For this review, take the finished solid that the model builds, in its own axes (mm). A direction names the side the tool comes from. Coordinates: 2 decimals unless noted, no trailing zeros. Order: outer loops, then holes, each group sorted by start corner. A loop starts at its lowest first (then second) coordinate and runs counter-clockwise, first axis right, second up. Notation, with made-up numbers: (76, 87) -> (115, 87) arc R23 cw to (115, 126) -> close; hole circle Ø9 at (44, 50). An arc over 180 degrees is marked (long way). Answer as a JSON object with one key per item and string values. Group by question number.
1) Draft analysis for pull direction X (two halves, no side actions). For faces 1 (the flat face through (790, -45, 250)), 2 (the cylindrical face through (-934.65, -36.38, 265.58)), 3 (the flat face through (-1130, -129, 25)), state which applies: +X half, -X half, draft (parallel to the pull), parting line (faces both ways), or undercut.
2) For pin 1 (23 mm diameter, centred on x = 1335, z = 424.71, fed in from +Y); pin 2 (15 mm diameter, centred on y = -172.5, z = 35, fed in from +X); pin 3 (10 mm diameter, centred on x = 96, y = -20.5, fed in from -Z); pin 4 (15 mm diameter, centred on y = -78, z = 15.5, fed in from -X), all flat-tipped, find the tip position at first contact; note any pin that passes through.
3) Add section A-A, the plane y = -141.5. Write out the cut boundary in (x, z).
4) Wall thickness on L1, parallel to Z at x = 1335, y = -260.25; L2, parallel to Y at x = 1092.5, z = 32; L3, parallel to Z at x = -1175, y = -262.25: over which ranges is each line inside the solid? List them lowest first.
5) Machinability: for faces 4 (the flat face through (1130, -126, 25)), 5 (the cylindrical face through (795.924, -31.007, 137.576)), 6 (the flat face through (1100, -154, 25)), 7 (the flat face through (-960, -45, 250)), 8 (the flat face through (-910, -45, 250)), which of the approach directions +Z, -Z, +X, -X, +Y, -Y give a long, thin tool a straight path to every point of the face, cutting with its end or side? Answer none if there is none.
6) Add section C-C, the plane x = -526. Write out the cut boundary in (y, z), then the cut area to 3 significant figures.
7) Add section B-B, the plane z = 168. Write out the cut boundary in (x, y).
from build123d import *

# Parameters (mm, degrees)
BOSS_EXTRUDE1_DEPTH = 50
SKETCH2_W           = 200
SKETCH2_H           = 20
BOSS_EXTRUDE2_DEPTH = 500
SKETCH4_R           = 20
BOSS_EXTRUDE3_DEPTH = 200
SKETCH6_R           = 30
SKETCH6_R_2         = 12
BOSS_EXTRUDE4_DEPTH = 25
SKETCH8_W           = 350
SKETCH8_H           = 20
BOSS_EXTRUDE5_DEPTH = 500
SKETCH9_R           = 20
CUT_EXTRUDE1_DEPTH  = 2356.175152722
LPATTERN2_COUNT     = 2
LPATTERN2_PITCH     = 1750
LPATTERN4_COUNT     = 2
LPATTERN4_PITCH     = 120
LPATTERN5_COUNT     = 2
LPATTERN5_PITCH     = 1600
CUT_EXTRUDE2_REACH  = 1488.01
SKETCH10_R          = 10
SKETCH11_R          = 10
CUT_EXTRUDE3_DEPTH  = 40


with BuildPart() as part:
    # Sketch1 → Boss-Extrude1 (new body)
    with BuildSketch(Plane.XY):
        Polygon((-1130, 0), (1130, 0), (1130, -255), (1100, -255), (1100, -50), (-1100, -50), (-1100, -255), (-1130, -255), align=None)
    extrude(amount=BOSS_EXTRUDE1_DEPTH)

    # Sketch2 → Boss-Extrude2 (add)
    with BuildSketch(Plane.XY):
        with Locations((-1125, -265)):
            Rectangle(SKETCH2_W, SKETCH2_H)
    extrude(amount=BOSS_EXTRUDE2_DEPTH)

    # Sketch4 → Boss-Extrude3 (add)
    with BuildSketch(Plane.XY.offset(50)):
        with Locations(Location((-935, -25, 0), (0, 0, 180))):
            Circle(SKETCH4_R)
    boss_extrude3 = extrude(amount=BOSS_EXTRUDE3_DEPTH)

    # Sketch6 → Boss-Extrude4 (add, symmetric)
    with BuildSketch(Plane(origin=(-935, 0, 0), x_dir=(0, -1, 0), z_dir=(-1, 0, 0))):
        with Locations(Location((25, 250, 0), (0, 0, 90))):
            Circle(SKETCH6_R)
        with Locations(Location((25, 250, 0), (0, 0, 90))):
            Circle(SKETCH6_R_2, mode=Mode.SUBTRACT)
    boss_extrude4 = extrude(amount=BOSS_EXTRUDE4_DEPTH, both=True)

    # Sketch8 → Boss-Extrude5 (add)
    with BuildSketch(Plane(origin=(0, 0, 0), x_dir=(-1, 0, 0), z_dir=(0, 0, -1))):
        with Locations((-1200, -265)):
            Rectangle(SKETCH8_W, SKETCH8_H)
    extrude(amount=-BOSS_EXTRUDE5_DEPTH)

    # Sketch9 → Cut-Extrude1 (cut, through all)
    with BuildSketch(Plane(origin=(-910, 0, 0), x_dir=(0, 0, -1), z_dir=(1, 0, 0))):
        with Locations((-249.707622987, -24.214075722)):
            Circle(SKETCH9_R)
    cut_extrude1 = extrude(amount=-CUT_EXTRUDE1_DEPTH, mode=Mode.SUBTRACT)

    # LPattern2: Boss-Extrude3, Boss-Extrude4, Cut-Extrude1 ×2
    with Locations(*[(i * LPATTERN2_PITCH, 0, 0) for i in range(1, LPATTERN2_COUNT)]):
        add(boss_extrude3)
        add(boss_extrude4)
        add(cut_extrude1, mode=Mode.SUBTRACT)

    # LPattern4: Boss-Extrude3, Boss-Extrude4, Cut-Extrude1 ×2
    with Locations(*[(i * LPATTERN4_PITCH, 0, 0) for i in range(1, LPATTERN4_COUNT)]):
        add(boss_extrude3)
        add(boss_extrude4)
        add(cut_extrude1, mode=Mode.SUBTRACT)

    # LPattern5: Boss-Extrude3, Boss-Extrude4, Cut-Extrude1 ×2
    with Locations(*[(i * LPATTERN5_PITCH, 0, 0) for i in range(1, LPATTERN5_COUNT)]):
        add(boss_extrude3)
        add(boss_extrude4)
        add(cut_extrude1, mode=Mode.SUBTRACT)

    # Sketch10 → Cut-Extrude2 (cut, up to next)
    with BuildSketch(Plane(origin=(0, -255, 0), x_dir=(1, 0, 0), z_dir=(0, 1, 0)), mode=Mode.PRIVATE) as cut_extrude2_sk1:
        with Locations(Location((1065, -424.7076, 0), (0, 0, 270))):
            Circle(SKETCH10_R)
    cut_extrude2_tool1 = extrude(cut_extrude2_sk1.sketch, amount=-CUT_EXTRUDE2_REACH, mode=Mode.PRIVATE) & part.part
    # Sketch10 → Cut-Extrude2 (cut, up to next)
    with BuildSketch(Plane(origin=(0, -255, 0), x_dir=(1, 0, 0), z_dir=(0, 1, 0)), mode=Mode.PRIVATE) as cut_extrude2_sk2:
        with Locations(Location((1065, -74.7076, 0), (0, 0, 270))):
            Circle(SKETCH10_R)
    cut_extrude2_tool2 = extrude(cut_extrude2_sk2.sketch, amount=-CUT_EXTRUDE2_REACH, mode=Mode.PRIVATE) & part.part
    # Sketch10 → Cut-Extrude2 (cut, up to next)
    with BuildSketch(Plane(origin=(0, -255, 0), x_dir=(1, 0, 0), z_dir=(0, 1, 0)), mode=Mode.PRIVATE) as cut_extrude2_sk3:
        with Locations(Location((1335, -424.7076, 0), (0, 0, 270))):
            Circle(SKETCH10_R)
    cut_extrude2_tool3 = extrude(cut_extrude2_sk3.sketch, amount=-CUT_EXTRUDE2_REACH, mode=Mode.PRIVATE) & part.part
    # Sketch10 → Cut-Extrude2 (cut, up to next)
    with BuildSketch(Plane(origin=(0, -255, 0), x_dir=(1, 0, 0), z_dir=(0, 1, 0)), mode=Mode.PRIVATE) as cut_extrude2_sk4:
        with Locations(Location((1335, -74.7076, 0), (0, 0, 270))):
            Circle(SKETCH10_R)
    cut_extrude2_tool4 = extrude(cut_extrude2_sk4.sketch, amount=-CUT_EXTRUDE2_REACH, mode=Mode.PRIVATE) & part.part
    # Sketch10 → Cut-Extrude2 (cut, up to next)
    with BuildSketch(Plane(origin=(0, -255, 0), x_dir=(1, 0, 0), z_dir=(0, 1, 0)), mode=Mode.PRIVATE) as cut_extrude2_sk5:
        with Locations(Location((-1175, -365.2924, 0), (0, 0, 270))):
            Circle(SKETCH10_R)
    cut_extrude2_tool5 = extrude(cut_extrude2_sk5.sketch, amount=-CUT_EXTRUDE2_REACH, mode=Mode.PRIVATE) & part.part
    # Sketch10 → Cut-Extrude2 (cut, up to next)
    with BuildSketch(Plane(origin=(0, -255, 0), x_dir=(1, 0, 0), z_dir=(0, 1, 0)), mode=Mode.PRIVATE) as cut_extrude2_sk6:
        with Locations(Location((-1055, -365.2924, 0), (0, 0, 270))):
            Circle(SKETCH10_R)
    cut_extrude2_tool6 = extrude(cut_extrude2_sk6.sketch, amount=-CUT_EXTRUDE2_REACH, mode=Mode.PRIVATE) & part.part
    # Sketch10 → Cut-Extrude2 (cut, up to next)
    with BuildSketch(Plane(origin=(0, -255, 0), x_dir=(1, 0, 0), z_dir=(0, 1, 0)), mode=Mode.PRIVATE) as cut_extrude2_sk7:
        with Locations(Location((-1175, -135.2924, 0), (0, 0, 270))):
            Circle(SKETCH10_R)
    cut_extrude2_tool7 = extrude(cut_extrude2_sk7.sketch, amount=-CUT_EXTRUDE2_REACH, mode=Mode.PRIVATE) & part.part
    # Sketch10 → Cut-Extrude2 (cut, up to next)
    with BuildSketch(Plane(origin=(0, -255, 0), x_dir=(1, 0, 0), z_dir=(0, 1, 0)), mode=Mode.PRIVATE) as cut_extrude2_sk8:
        with Locations(Location((-1055, -135.2924, 0), (0, 0, 270))):
            Circle(SKETCH10_R)
    cut_extrude2_tool8 = extrude(cut_extrude2_sk8.sketch, amount=-CUT_EXTRUDE2_REACH, mode=Mode.PRIVATE) & part.part
    add(cut_extrude2_tool1.solids().sort_by_distance((1065, -255, 424.7076))[0], mode=Mode.SUBTRACT)
    add(cut_extrude2_tool2.solids().sort_by_distance((1065, -255, 74.7076))[0], mode=Mode.SUBTRACT)
    add(cut_extrude2_tool3.solids().sort_by_distance((1335, -255, 424.7076))[0], mode=Mode.SUBTRACT)
    add(cut_extrude2_tool4.solids().sort_by_distance((1335, -255, 74.7076))[0], mode=Mode.SUBTRACT)
    add(cut_extrude2_tool5.solids().sort_by_distance((-1175, -255, 365.2924))[0], mode=Mode.SUBTRACT)
    add(cut_extrude2_tool6.solids().sort_by_distance((-1055, -255, 365.2924))[0], mode=Mode.SUBTRACT)
    add(cut_extrude2_tool7.solids().sort_by_distance((-1175, -255, 135.2924))[0], mode=Mode.SUBTRACT)
    add(cut_extrude2_tool8.solids().sort_by_distance((-1055, -255, 135.2924))[0], mode=Mode.SUBTRACT)

    # Sketch11 → Cut-Extrude3 (cut)
    with BuildSketch(Plane(origin=(0, 0, 0), x_dir=(-1, 0, 0), z_dir=(0, 0, -1))):
        with Locations((-100, -25)):
            Circle(SKETCH11_R)
    extrude(amount=-CUT_EXTRUDE3_DEPTH, mode=Mode.SUBTRACT)


solid = part.part
Output values:
{
 "1": {"face 1": "undercut", "face 2": "draft", "face 3": "-X half"},
 "2": {"pin 1": "stops at y = -255", "pin 2": "stops at x = 1130", "pin 3": "stops at z = 0", "pin 4": "stops at x = -1130"},
 "3": {"outline": "(-1130, 0) -> (-1100, 0) -> (-1100, 50) -> (-1130, 50) -> close; (1100, 0) -> (1130, 0) -> (1130, 50) -> (1100, 50) -> close"},
 "4": {"L1": "z = 0 to 64.71, 84.71 to 414.71, 434.71 to 500", "L2": "y = -275 to -255, -50 to 0", "L3": "z = 0 to 125.29, 145.29 to 355.29, 375.29 to 500"},
 "5": {"face 4": "+Z, -Z, +X, +Y", "face 5": "none", "face 6": "+Z, -Z", "face 7": "+Z, -X, +Y, -Y", "face 8": "+Z, +Y, -Y"},
 "6": {"outline": "(-50, 0) -> (0, 0) -> (0, 50) -> (-50, 50) -> close", "area": "2,500 mm²"},
 "7": {"outline": "(-1225, -275) -> (-1025, -275) -> (-1025, -255) -> (-1225, -255) -> close; circle Ø40 at (-935, -25); circle Ø40 at (-815, -25); circle Ø40 at (665, -25); circle Ø40 at (815, -25); (1025, -275) -> (1375, -275) -> (1375, -255) -> (1025, -255) -> close"}
}
